```python
from build123d import *

# Parameters (mm, degrees)
BOSS_EXTRUDE1_OUTLINE_R = 3.556
BOSS_EXTRUDE1_OUTLINE_W = 260.9469
BOSS_EXTRUDE1_OUTLINE_H = 138.1252
BOSS_EXTRUDE1_DEPTH     = 76.2
CUT_EXTRUDE1_DEPTH      = 355.32482824
CUT_EXTRUDE1_DEPTH_BACK = 355.32482824
FILLET1_R               = 2.54
SKETCH7_W               = 260.9469
SKETCH7_H               = 22.1996
CUT_EXTRUDE2_DEPTH      = 347.152897849
FILLET2_R               = 6.35
SKETCH8_W               = 190.775627824
SKETCH8_H               = 235.521960295
CUT_EXTRUDE4_DEPTH      = 347.144751077
SKETCH9_W               = 165.75862987
SKETCH9_H               = 108.368614936
CUT_EXTRUDE5_DEPTH      = 227.747805823


# Read off the part's stored shape, not the designer's step: Boss-Extrude1
with BuildPart() as part:
    # Boss-Extrude1 outline → Boss-Extrude1 (new body)
    with BuildSketch(Plane.XY):
        with BuildLine():
            Line((-286.3596, -22.225), (9.525, -22.225))
            ThreePointArc((9.525, -22.225), (19.05, -12.7), (9.525, -3.175))
            ThreePointArc((9.525, -3.175), (19.05, 6.35), (9.525, 15.875))
            ThreePointArc((9.525, 15.875), (2.789807909, 18.664807909), (0, 25.4))
            Line((0, 25.4), (0, 131.7752))
            ThreePointArc((0, 131.7752), (2.789807909, 138.510392091), (9.525, 141.3002))
            ThreePointArc((9.525, 141.3002), (19.05, 150.8252), (9.525, 160.3502))
            ThreePointArc((9.525, 160.3502), (19.05, 169.8752), (9.525, 179.4002))
            Line((9.525, 179.4002), (-6.35, 179.4002))
            Line((-6.35, 179.4002), (-6.35, 163.5252))
            Line((-6.35, 163.5252), (-7.9502, 163.5252))
            Line((-7.9502, 163.5252), (-7.9502, 160.3502))
            Line((-7.9502, 160.3502), (-268.9098, 160.3502))
            Line((-268.9098, 160.3502), (-268.9098, 163.5252))
            Line((-268.9098, 163.5252), (-270.51, 163.5252))
            Line((-270.51, 163.5252), (-270.51, 179.4002))
            Line((-270.51, 179.4002), (-286.385, 179.4002))
            ThreePointArc((-286.385, 179.4002), (-295.91, 169.8752), (-286.385, 160.3502))
            ThreePointArc((-286.385, 160.3502), (-295.897297883, 150.818850004), (-286.3723, 141.3002))
            ThreePointArc((-286.3723, 141.3002), (-279.637107909, 138.510392091), (-276.8473, 131.7752))
            Line((-276.8473, 131.7752), (-276.8473, 25.4))
            ThreePointArc((-276.8473, 25.4), (-279.637107909, 18.664807909), (-286.3723, 15.875))
            ThreePointArc((-286.3723, 15.875), (-295.8973, 6.35), (-286.3723, -3.175))
            ThreePointArc((-286.3723, -3.175), (-295.884597883, -12.706349996), (-286.3596, -22.225))
        make_face()
        with Locations((-286.3596, -12.7)):
            Circle(BOSS_EXTRUDE1_OUTLINE_R, mode=Mode.SUBTRACT)
        with Locations((-286.3723, 6.35)):
            Circle(BOSS_EXTRUDE1_OUTLINE_R, mode=Mode.SUBTRACT)
        with Locations((9.525, -12.7)):
            Circle(BOSS_EXTRUDE1_OUTLINE_R, mode=Mode.SUBTRACT)
        with Locations((9.525, 6.35)):
            Circle(BOSS_EXTRUDE1_OUTLINE_R, mode=Mode.SUBTRACT)
        with Locations((-286.3723, 150.8252)):
            Circle(BOSS_EXTRUDE1_OUTLINE_R, mode=Mode.SUBTRACT)
        with Locations((-286.385, 169.8752)):
            Circle(BOSS_EXTRUDE1_OUTLINE_R, mode=Mode.SUBTRACT)
        with Locations((-138.42365, 78.5876)):
            Rectangle(BOSS_EXTRUDE1_OUTLINE_W, BOSS_EXTRUDE1_OUTLINE_H, mode=Mode.SUBTRACT)
        with Locations((9.525, 150.8252)):
            Circle(BOSS_EXTRUDE1_OUTLINE_R, mode=Mode.SUBTRACT)
        with Locations((9.525, 169.8752)):
            Circle(BOSS_EXTRUDE1_OUTLINE_R, mode=Mode.SUBTRACT)
    extrude(amount=BOSS_EXTRUDE1_DEPTH)

    # Sketch5 → Cut-Extrude1 (cut, two sides: drawn at the far end of the back side and taken through both)
    with BuildSketch(Plane.ZY.offset(276.8473).offset(-CUT_EXTRUDE1_DEPTH_BACK)):
        Polygon((1.6002, -22.225), (8.641107133, 179.4002), (76.2, 179.4002), (76.2, -22.225), align=None)
    extrude(amount=CUT_EXTRUDE1_DEPTH + CUT_EXTRUDE1_DEPTH_BACK, mode=Mode.SUBTRACT)

    # Fillet1
    fillet1_edges = [part.edges().sort_by_distance(p)[0] for p in [
        (-286.385, 160.3502, 3.987933237),
        (-286.3723, -3.175, 1.132720329),
        (9.525, -3.175, 1.132720329),
        (9.525, 160.3502, 3.987933237),
    ]]
    fillet(fillet1_edges, radius=FILLET1_R)

    # Sketch7 → Cut-Extrude2 (cut, through all)
    with BuildSketch(Plane(origin=(0, 0, 0), x_dir=(-1, 0, 0), z_dir=(0, 0, -1))):
        with Locations((138.42365, -6.35)):
            Rectangle(SKETCH7_W, SKETCH7_H)
    extrude(amount=-CUT_EXTRUDE2_DEPTH, mode=Mode.SUBTRACT)

    # Fillet2
    fillet2_edges = [part.edges().sort_by_distance(p)[0] for p in [
        (-268.8971, 4.7498, 1.271090386),
        (-268.8971, -17.4498, 0.883476829),
        (-7.9502, -17.4498, 0.883476829),
        (-7.9502, 4.7498, 1.271090386),
    ]]
    fillet(fillet2_edges, radius=FILLET2_R)

    # Sketch8 → Cut-Extrude4 (cut, through all)
    with BuildSketch(Plane(origin=(0, -0.082881646, 2.373419811), x_dir=(1, 0, 0), z_dir=(0, -0.03489949670250444, 0.9993908270190958))):
        with Locations((-233.811463912, 74.917246318)):
            Rectangle(SKETCH8_W, SKETCH8_H)
    extrude(amount=-CUT_EXTRUDE4_DEPTH, mode=Mode.SUBTRACT)

    # Sketch9 → Cut-Extrude5 (cut, through all)
    with BuildSketch(Plane(origin=(0, -0.082881646, 2.373419811), x_dir=(1, 0, 0), z_dir=(0, -0.03489949670250444, 0.9993908270190958))):
        with Locations((-55.544335065, 24.534127322)):
            Rectangle(SKETCH9_W, SKETCH9_H)
    extrude(amount=-CUT_EXTRUDE5_DEPTH, mode=Mode.SUBTRACT)


solid = part.part
```
Here's how the part is built. I have some questions about the finished solid (model axes, mm). A direction names the side the tool comes from. Round coordinates to 2 decimals unless told otherwise and drop trailing zeros. Write each loop counter-clockwise with the first axis right and the second up, starting at its lowest first coordinate (ties: lowest second). Pieces come first, ordered by that corner, then holes.
Q1. If we mould it in two halves opening along Y, with no side actions, what happens to faces 6 (the flat face through (-7.95, 162, 4)), 7 (the cylindrical face through (18.587, 172.809, 4.26)), 8 (the flat face through (-74, 147.65, 4)), 9 (the cylindrical face through (8.754, 166.404, 4.17))? For each: +Y half, -Y half, draft (parallel to the pull), parting line (faces both ways), or undercut.
Q2. Please list where these lines run through material, in increasing order: probe 1 along Y at (x, z) = (12, 4.75); probe 2 along X at (y, z) = (86, 4.5); probe 3 along Y at (x, z) = (-80, 4.5).
Q3. If we section it at C-C on y = 87: Write out the boundary of the cut face in (x, z).
Q4. If we section it at A-A on x = -23: Write out the boundary of the cut face in (y, z).
Q5. If we section it at B-B on z = 1.75: Give the number of separate pieces and of enclosed holes in the cut face, plus the area to 3 significant figures.
Q6. Which directions (+Z, -Z, +X, -X, +Y, -Y) give clear straight access to the entire face, cutting with the end or side of a thin tool? Please do faces 1 (the flat face through (-72, 160.35, 4)), 2 (the flat face through (0, 105, 3)), 3 (the flat face through (-138.424, 154, 4)), 4 (the flat face through (-7.95, 113, 3)), 5 (the flat face through (-43, 152, 0)).
Q7. Will these pins go through, and if not, where does the flat tip stop? P1, Ø2, axis at x = -66.5, z = 5, coming from the +Y side; P2, Ø1, axis at x = -7.5, z = 4.5, coming from the -Y side; P3, Ø4, axis at x = -92, z = 4, coming from the -Y side.
Answer below:
1. face 6: draft
1. face 7: undercut
1. face 8: -Y half
1. face 9: undercut
2. probe 1: y = 141.63 to 148.27, 153.38 to 167.32, 172.43 to 179.07
2. probe 2: x = -7.95 to 0
2. probe 3: y = 147.65 to 160.35
3. outline: (-7.95, 0) - (0, 0) - (0, 5.41) - (-7.95, 5.41) - close
4. outline: (147.65, 0) - (160.35, 0) - (160.35, 7.98) - (147.65, 7.53) - close
5. separate pieces: 1
5. enclosed holes: 2
5. area: 3,020 mm2
6. face 1: +Z, -Z, -X, +Y
6. face 2: +Z, -Z, +X, -Y
6. face 3: +Z, -Z, -X, +Y, -Y
6. face 4: +Z, -Z, -X, -Y
6. face 5: -Z, +X, -X, +Y, -Y
7. P1: stops at y = 160.35
7. P2: stops at y = 78.59
7. P3: stops at y = 147.65
